Design review of the part built by this model. Coordinates are the model's own, in mm. A direction names the side the tool comes from. Give positions to 0.01 mm unless a question says otherwise; leave off trailing zeros. Order: outer loops, then holes, each group sorted by start corner. A loop starts at its lowest first (then second) coordinate and runs counter-clockwise, first axis right, second up. Notation, with made-up numbers: M 28.25,22.5 L 59.25,22.5 A35 ccw 59.25,60.5 Z; hole C -30,5.25 d8. An arc over 180 degrees is marked long. Answer as a JSON object with one key per item and string values.
from build123d import *


with BuildPart() as part:
    # Sketch2 → Revolve1 (revolve)
    with BuildSketch(Plane.XY):
        with BuildLine():
            Line((24, 7.15), (24, 6.5))
            Line((24, 6.5), (23, 6.5))
            Line((23, 6.5), (23, 6.8))
            Line((23, 6.8), (22, 6.8))
            Line((22, 6.8), (22, 5.5))
            Line((22, 5.5), (2, 5.5))
            Line((2, 5.5), (2, 6.8))
            Line((2, 6.8), (1, 6.8))
            Line((1, 6.8), (1, 6.5))
            Line((1, 6.5), (0, 6.5))
            Line((0, 6.5), (0, 7.15))
            ThreePointArc((0, 7.15), (0.102512627, 7.397487373), (0.35, 7.5))
            Line((0.35, 7.5), (3.25, 7.5))
            Line((3.25, 7.5), (3.25, 7.15))
            Line((3.25, 7.15), (4.35, 7.15))
            Line((4.35, 7.15), (4.35, 7.5))
            Line((4.35, 7.5), (19.65, 7.5))
            Line((19.65, 7.5), (19.65, 7.15))
            Line((19.65, 7.15), (20.75, 7.15))
            Line((20.75, 7.15), (20.75, 7.5))
            Line((20.75, 7.5), (23.65, 7.5))
            ThreePointArc((23.65, 7.5), (23.897487373, 7.397487373), (24, 7.15))
        make_face()
    revolve(axis=Axis((0, 0, 0), (1, 0, 0)))


solid = part.part
(1) To check wall thickness, follow L1, parallel to Z at x = 22.5, y = 0; L2, parallel to Z at x = 19.75, y = -0.25; L3, parallel to X at y = -1, z = -6. State the ranges of each line that lie inside material, in increasing order. Write a range as from..to.
Checked values:
{"L1": "z = -7.5..-6.8, 6.8..7.5", "L2": "z = -7.15..-5.49, 5.49..7.15", "L3": "x = 2..22"}
(2) We need section B-B (x = 1.5). Write out the cut boundary in (y, z).
Checked values:
{"outline": "C 0,0 d15; hole C 0,0 d13.6"}
(3) We need section A-A (x = 17). Write out the cut boundary in (y, z), plus the area to 3 significant figures.
Checked values:
{"outline": "C 0,0 d15; hole C 0,0 d11", "area": "81.7 mm^2"}
(4) Insertion check: pin 1 (1.5 mm diameter, centred on x = 21, y = -6, fed in from -Z); pin 2 (7.5 mm diameter, centred on y = -3.5, z = 2, fed in from -X); pin 3 (4.5 mm diameter, centred on y = -0.5, z = 1, fed in from -X); pin 4 (3 mm diameter, centred on y = 4, z = -1, fed in from +X). Each pin has a flat end and moves straight along its axis. Give the tip position at first contact, or say it passes through.
Checked values:
{"pin 1": "stops at z = -5.36", "pin 2": "stops at x = 0", "pin 3": "passes through", "pin 4": "stops at x = 22"}
(5) Tool access review of faces 4 (the flat face through (2, -6, 0)), 5 (the cylindrical face through (11.86, -1.19, -5.37)), 6 (the cylindrical face through (23.493, -5.158, -3.955)): name each direction out of +Z, -Z, +X, -X, +Y, -Y from which nothing blocks a thin tool from reaching the whole face with its end or side.
Checked values:
{"face 4": "none", "face 5": "+X, -X", "face 6": "+X"}
(6) Draft analysis for pull direction Z (two halves, no side actions). For faces 1 (the cylindrical face through (20.21, -0.93, 7.09)), 2 (the flat face through (22, 6, 0)), 3 (the flat face through (24, 3, -6)), state which applies: +Z half, -Z half, draft (parallel to the pull), parting line (faces both ways), or undercut.
Checked values:
{"face 1": "parting line", "face 2": "undercut", "face 3": "draft"}
